Check sheet for the drawn part. Datum: minimum x, y, z corner. Units: mm. Coordinates: 2 decimals unless noted, no trailing zeros. Order: outer loops, then holes, each group sorted by start corner. A loop starts at its lowest first (then second) coordinate and runs counter-clockwise, first axis right, second up. Notation, with made-up numbers: M 39.25,11.5 L 45.25,11.5 A20 cw 45.25,49.5 Z; hole C -6.5,-31 d1. An arc over 180 degrees is marked long. Use one line per item in the form item = value. Start each with the question number.
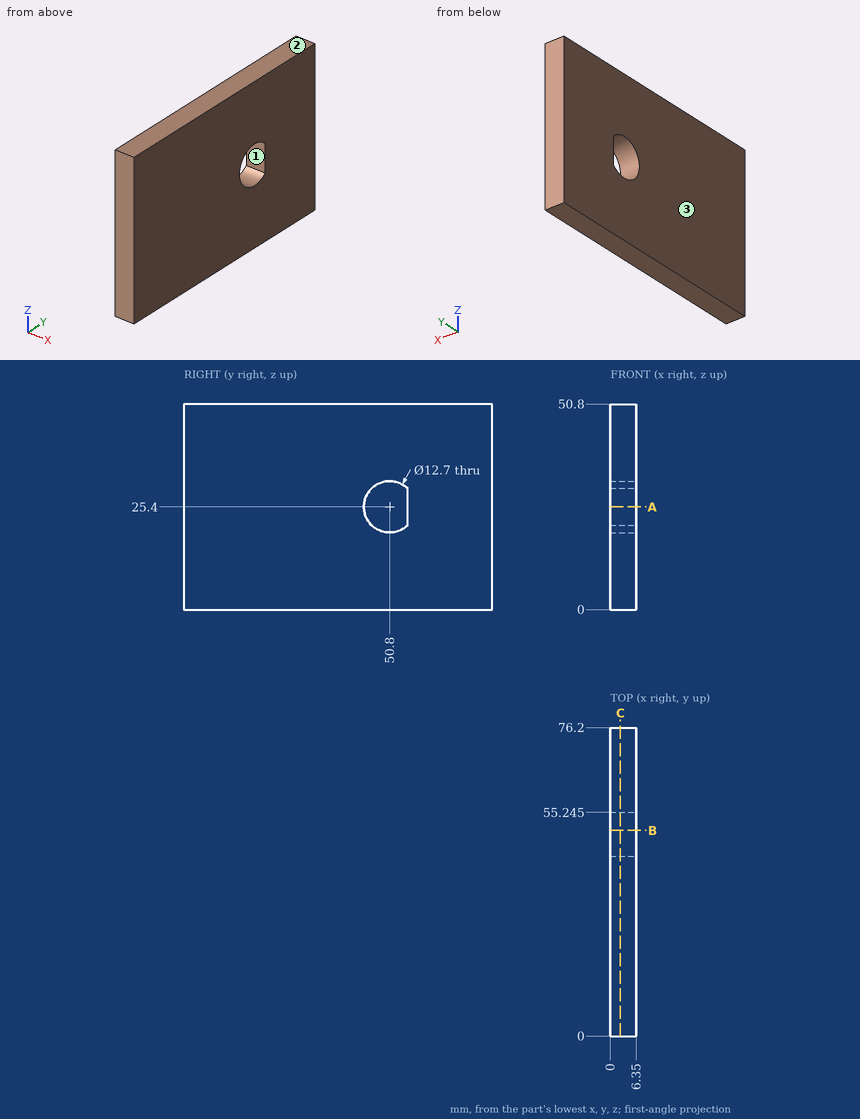
1. Cross-section at C-C on x = 2.5. Enter the section's corners in (y, z) (3 decimals).
2. Release check for a two-part mould opening along Z. For the marked faces 1, 2 and 3 record: pulls with the +Z half, pulls with the -Z half, needs draft (parallel to the pull), parting line crosses it, or undercut.
3. Material ranges on line 1 along Z through (x, y) = (2, 50.8); line 2 along Y through (x, z) = (2.5, 25.4) (3 decimals); line 3 along Z through (x, y) = (5, 53), recorded low to high.
4. Cross-section at B-B on y = 50.8. Enter the section's corners in (x, z), and give its area (3 significant figures).
5. Cross-section at A-A on z = 25.4. Enter the section's corners in (x, y) (3 decimals), and give its area (3 significant figures).
Final values:
q1.outline = M 0,0 L 76.2,0 L 76.2,50.8 L 0,50.8 Z; hole M 55.245,20.865 L 55.245,29.935 A6.35 ccw long Z
q2.face_1 = undercut
q2.face_2 = pulls with the +Z half
q2.face_3 = needs draft
q3.line_1 = 0 to 19.05, 31.75 to 50.8
q3.line_2 = 0 to 44.45, 55.245 to 76.2
q3.line_3 = 0 to 19.44, 31.36 to 50.8
q4.outline = M 0,0 L 6.35,0 L 6.35,19.05 L 0,19.05 Z; M 0,31.75 L 6.35,31.75 L 6.35,50.8 L 0,50.8 Z
q4.area = 242 mm2
q5.outline = M 0,0 L 6.35,0 L 6.35,44.45 L 0,44.45 Z; M 0,55.245 L 6.35,55.245 L 6.35,76.2 L 0,76.2 Z
q5.area = 415 mm2
